Autodesk Inventor part; units mm, degrees
ref_plane "YZ Plane" through (0, 0, 0) normal (1, 0, 0) x (0, 1, 0)
ref_plane "XZ Plane" through (0, 0, 0) normal (0, 1, 0) x (-1, 0, 0)
ref_plane "XY Plane" through (0, 0, 0) normal (0, 0, 1) x (1, 0, 0)
sketch "Sketch1" plane through (0, 0, 0) normal (0, 0, 1) x (1, 0, 0)
  line L0 (0, 0) -> (25, 0)
  line L1 (25, 0) -> (25, 40)
  line L2 (25, 40) -> (0, 40)
  line L3 (0, 40) -> (0, 0)
  dimension "d1" = 25
  dimension "d2" = 40
  dimension "d3" = 25
extrude "Extrusion1" add sketch "Sketch1" against normal blind 30
sketch "Sketch2" plane through (25, 0, 0) normal (1, 0, 0) x (0, 0, -1)
  line L0 (0, 0) -> (30, 0)
  circle A0 centre (15, 6.56) radius 2.46
extrude "Extrusion2" cut sketch "Sketch2" against normal blind 30
sketch "Sketch3" plane through (0, 0, 0) normal (-1, 0, 0) x (0, 0, 1)
  line L0 (0, 0) -> (-30, 0)
  line L1 (-25.05, 0) -> (-4.95, 0)
  line L2 (-4.95, 0) -> (-4.95, 33.12)
  line L3 (-4.95, 33.12) -> (-25.05, 33.12)
  line L4 (-25.05, 33.12) -> (-25.05, 0)
  dimension "d11" = 20.1
extrude "Extrusion3" cut sketch "Sketch3" against normal blind 20
sketch "Sketch4" plane through (0, 0, 0) normal (0, -1, 0) x (1, 0, 0)
  line L0 (20, -4.95) -> (20, -25.05)
  line L1 (20, -15) -> (25, -15)
  line L2 (25, 0) -> (25, -30)
  line L3 (20, -8.025) -> (25, -8.025)
  line L4 (25, -8.025) -> (25, -21.975)
  line L5 (25, -21.975) -> (20, -21.975)
  line L6 (20, -21.975) -> (20, -8.025)
  line L7 (20, -8.025) -> (25, -21.975) construction
  line L8 (25, -8.025) -> (20, -21.975) construction
  line L9 (25, -12.54) -> (25, -17.46)
  point P0 (0, 0)
  point P1 (22.5, -15)
  dimension "d14" = 13.95
extrude "Extrusion4" add sketch "Sketch4" along normal blind 15
sketch "Sketch5" plane through (20, 0, 0) normal (-1, 0, 0) x (0, 0, 1)
  circle A0 centre (-15, 6.56) radius 2.46
  circle A1 centre (-15, 6.56) radius 4.7025
  circle A2 centre (-15, 6.56) radius 2.46
  circle A3 centre (-15, 6.56) radius 2.46
  point P0 (0, 0)
  dimension "d17" = 9.405
extrude "Extrusion5" cut sketch "Sketch5" against normal blind 2.1
sketch "Sketch6" plane through (25, 0, 0) normal (1, 0, 0) x (0, 0, -1)
  circle A0 centre (15, 6.56) radius 4.7025
  line L0 (15, 6.56) -> (15, 23.56)
  circle A1 centre (15, 23.56) radius 2.46
  point P0 (0, 0)
  dimension "d20" = 17
  dimension "d21" = 4.92
extrude "Extrusion6" cut sketch "Sketch6" against normal blind 10 contours A1
sketch "Sketch7" plane through (20, 0, 0) normal (-1, 0, 0) x (0, 0, 1)
  circle A0 centre (-15, 23.56) radius 2.46
  circle A1 centre (-15, 23.56) radius 4.7025
  point P0 (0, 0)
  dimension "d24" = 9.405
extrude "Extrusion7" cut sketch "Sketch7" against normal blind 2.1
sketch "Sketch9" plane through (25, 0, 0) normal (1, 0, 0) x (0, 0, -1)
  circle A0 centre (15, 6.56) radius 2.46
  circle A1 centre (15, 6.56) radius 2.46
  circle A2 centre (15, 23.56) radius 2.46
  circle A3 centre (15, 23.56) radius 2.46
  line L0 (30, 40) -> (30, 0)
  line L1 (30, 0) -> (30, 40)
  line L2 (30, 40) -> (0, 40)
  line L3 (0, 40) -> (0, 0)
  line L4 (0, 0) -> (8.025, 0)
  line L5 (21.975, 0) -> (21.975, -15)
  line L6 (21.975, -15) -> (8.025, -15)
  line L7 (8.025, -15) -> (8.025, 0)
  line L8 (0, 0) -> (8.025, 0)
  line L9 (21.975, 0) -> (30, 0)
extrude "Extrusion8" add sketch "Sketch9" along normal blind 5
sketch "Sketch10" plane through (0, 40, 0) normal (0, 1, 0) x (1, 0, 0)
  line L0 (0, 30) -> (30, 30)
  line L1 (30, 0) -> (0, 0)
  line L2 (0, 30) -> (30, 30)
  line L3 (30, 30) -> (30, 0)
  line L4 (30, 0) -> (0, 0)
  line L5 (0, 0) -> (0, 30)
extrude "Extrusion9" add sketch "Sketch10" along normal blind 30
sketch "Sketch12" plane through (30, 0, 0) normal (1, 0, 0) x (0, 0, -1)
  circle A0 centre (15, 6.56) radius 2.46
  line L0 (15, 6.56) -> (15, 15.06)
  circle A1 centre (15, 15.06) radius 2.525
  point P0 (0, 0)
  dimension "d31" = 8.5
  dimension "d33" = 5.05
extrude "Extrusion10" cut sketch "Sketch12" against normal blind 30 contours A1
sketch "Sketch14" plane through (0, 0, 0) normal (0, 0, 1) x (1, 0, 0)
  line L0 (30, 70) -> (0, 70)
  line L1 (0, 70) -> (0, 85)
  line L2 (-15, 100) -> (-23, 100)
  line L3 (30, 0) -> (30, 70)
  line L4 (30, 118) -> (30, 70)
  arc A0 (0, 85) -> (-15, 100) centre (-15, 85) ccw
  line L5 (30, 105) -> (30, 100)
  line L6 (-18, 134) -> (-23, 136)
  line L7 (-18, 102) -> (-23, 100)
  line L8 (-18, 102) -> (-13, 118)
  line L9 (-13, 118) -> (-18, 134)
  line L10 (15, 136) -> (30, 118)
  line L11 (-23, 136) -> (15, 136)
  point P0 (0, 0)
  point P1 (0, 100)
  dimension "d47" = 30
  dimension "d54" = 15
extrude "Extrusion12" add sketch "Sketch14" against normal blind 30
sketch "Sketch15" plane through (0, 0, -25.05) normal (-1, 0, 0) x (0, 0, 1)
  line L0 (0, 33.12) -> (20.1, 33.12)
  line L1 (20.1, 33.12) -> (20.1, 0)
  line L2 (0, 33.12) -> (20.1, 33.12)
  line L3 (20.1, 33.12) -> (20.1, 31.1)
  line L4 (20.1, 31.1) -> (0, 31.1)
  line L5 (0, 31.1) -> (0, 33.12)
  point P0 (25.05, 0)
  dimension "d57" = 2.02
extrude "Extrusion13" add sketch "Sketch15" against normal blind 20
properties part number "rec_a_32mm_x_30mm"
Can you work these out from the model? Positions are in its coordinate system, mm. A direction names the side the tool comes from. Coordinates: 2 decimals unless noted, no trailing zeros. Loops run counter-clockwise (first coordinate to the right, second up) from the corner with the lowest first, then second, coordinate; pieces in that order, holes last.
Item 1: Suppose I cut it at A-A (y = 6.56). Please give me the cut outline in (x, z).
Answers below:
outline: (0, -30) - (30, -30) - (30, -17.46) - (22.1, -17.46) - (22.1, -19.7) - (20, -19.7) - (20, -25.05) - (0, -25.05) - close; (0, -4.95) - (20, -4.95) - (20, -10.3) - (22.1, -10.3) - (22.1, -12.54) - (30, -12.54) - (30, 0) - (0, 0) - close
Item 2: Which directions (+Z, -Z, +X, -X, +Y, -Y) give clear straight access to the entire face, cutting with the end or side of a thin tool? Please do faces 1 (the face through (10, 31.1, -15)), 2 (the face through (18, 0, -27)), 3 (the face through (25, -8, -8.025)), 4 (the face through (-20.5, 101, -14.8)), 5 (the face through (22.1, 4.5, -13)).
Answers below:
face 1: -X, -Y
face 2: -Z, +X, -X, -Y
face 3: +Z, +X, -X, -Y
face 4: +Z, -Z, -X
face 5: -X
Item 3: Please list where these lines run through material, in increasing order: L1, parallel to Z at x = 23, y = 15; L2, parallel to Y at x = 24, z = -15 (3 decimals); L3, parallel to X at y = -1, z = -13.25.
Answers below:
L1: z = -30 to -17.52, -12.48 to 0
L2: y = -15 to 4.1, 9.02 to 12.535, 17.585 to 21.1, 26.02 to 125.2
L3: x = 20 to 30
Item 4: Suppose I cut it at C-C (x = 8). Please give me the cut outline in (y, z), then the cut area to 3 significant figures.
Answers below:
outline: (0, -30) - (136, -30) - (136, 0) - (0, 0) - (0, -4.95) - (31.1, -4.95) - (31.1, -25.05) - (0, -25.05) - close
area: 3,450 mm2
Item 5: If we mould it in two halves opening along Z, with no side actions, what happens to faces 6 (the face through (15, 0, -3)), 7 (the face through (10, 16, -25.05)), 8 (the face through (9, 69, 0))? For each: released by +Z, released by -Z, zero draft, split by the parting line, or undercut.
Answers below:
face 6: zero draft
face 7: undercut
face 8: released by +Z
Item 6: I'm going to push flat-ended pins straight in: pin 1 (7.5 mm diameter, centred on y = 23.5, z = -14.5, fed in from -X); pin 2 (10 mm diameter, centred on y = 118, z = -15, fed in from -X); pin 3 (6.5 mm diameter, centred on x = -19.5, z = -19, fed in from -Y). Where does each tip first touch, or does it pass through?
Answers below:
pin 1: stops at x = 22.1
pin 2: stops at x = -14.56
pin 3: stops at y = 100
Item 7: Suppose I cut it at B-B (z = -15). State how many separate pieces and enclosed holes the cut face has, then the cut area to 3 significant figures.
Answers below:
separate pieces: 4
enclosed holes: 0
area: 3,930 mm2
Item 8: Suppose I cut it at D-D (y = 36). Please give me the cut outline in (x, z), then the cut area to 3 significant figures.
Answers below:
outline: (0, -30) - (30, -30) - (30, 0) - (0, 0) - close
area: 900 mm2
